Design review of the part built by this model. Coordinates are the model's own, in mm. Round coordinates to 2 decimals unless told otherwise and drop trailing zeros. Order: outer loops, then holes, each group sorted by start corner. A loop starts at its lowest first (then second) coordinate and runs counter-clockwise, first axis right, second up. Notation, with made-up numbers: M 32,-5.5 L 38,-5.5 A31 cw 38,25.5 Z; hole C -9,-34.5 d6. An arc over 180 degrees is marked long. Write each question's results on one line, items separated by ' | '. Start each with the question number.
Item 1: Wall thickness on line 1 (Z direction, x = -36, y = 0.55); line 2 (X direction, y = 0.5, z = -32); line 3 (Z direction, x = 43.5, y = 0.9): over which ranges is each line inside the solid? List them lowest first. Write a range as [from, to].
Item 2: Take a section at C-C, the plane y = 1.15. Count the separate pieces of the cut face and the enclosed holes in it, plus the area to 3 significant figures.
Item 3: Take a section at B-B, the plane z = 11.5. Write out the cut boundary in (x, y), plus the area to 3 significant figures.
Item 4: Take a section at A-A, the plane x = 43.5. Write out the cut boundary in (y, z), plus the area to 3 significant figures.
```python
from build123d import *

# Parameters (mm, degrees)
BOSS_EXTRUDE1_DEPTH = 2.3
SKETCH2_R           = 1
CUT_EXTRUDE1_DEPTH  = 2.3
SKETCH3_W           = 10
SKETCH3_H           = 2.3
CUT_EXTRUDE2_DEPTH  = 2.3
SKETCH4_W           = 15
SKETCH4_H           = 4
CUT_EXTRUDE3_DEPTH  = 10
SKETCH5_W           = 2.3
SKETCH5_H           = 10
CUT_EXTRUDE4_DEPTH  = 2.3
FILLET1_R           = 1
SKETCH6_W           = 4
SKETCH6_H           = 15
SKETCH6_W_2         = 10
SKETCH6_H_2         = 4
CUT_EXTRUDE5_DEPTH  = 10
FILLET3_R           = 1
SKETCH7_R           = 3
CUT_EXTRUDE6_DEPTH  = 10


with BuildPart() as part:
    # Sketch1 → Boss-Extrude1 (new body)
    with BuildSketch(Plane(origin=(0, 0, 0), x_dir=(1, 0, 0), z_dir=(0, 1, 0))):
        Polygon((0, -50), (-49.5, -50), (-49.5, 0), (-49.5, 35), (0, 35), (49.5, 35), (49.5, 0), (49.5, -50), align=None)
    extrude(amount=BOSS_EXTRUDE1_DEPTH)

    # Sketch2 → Cut-Extrude1 (cut)
    with BuildSketch(Plane(origin=(0, 2.3, 0), x_dir=(1, 0, 0), z_dir=(0, 1, 0))):
        with Locations((-20, 32)):
            Circle(SKETCH2_R)
        with Locations((20, 32)):
            Circle(SKETCH2_R)
    extrude(amount=-CUT_EXTRUDE1_DEPTH, mode=Mode.SUBTRACT)

    # Sketch3 → Cut-Extrude2 (cut)
    with BuildSketch(Plane(origin=(0, 2.3, 0), x_dir=(1, 0, 0), z_dir=(0, 1, 0))):
        with Locations((-15, -43.85)):
            Rectangle(SKETCH3_W, SKETCH3_H)
        with Locations((15, -43.85)):
            Rectangle(SKETCH3_W, SKETCH3_H)
    extrude(amount=-CUT_EXTRUDE2_DEPTH, mode=Mode.SUBTRACT)

    # Sketch4 → Cut-Extrude3 (cut)
    with BuildSketch(Plane(origin=(0, 2.3, 0), x_dir=(1, 0, 0), z_dir=(0, 1, 0))):
        with Locations((-17.5, 25)):
            Rectangle(SKETCH4_W, SKETCH4_H)
        with Locations((17.5, 25)):
            Rectangle(SKETCH4_W, SKETCH4_H)
    extrude(amount=-CUT_EXTRUDE3_DEPTH, mode=Mode.SUBTRACT)

    # Sketch5 → Cut-Extrude4 (cut)
    with BuildSketch(Plane(origin=(0, 2.3, 0), x_dir=(1, 0, 0), z_dir=(0, 1, 0))):
        with Locations((-36.15, 7.5)):
            Rectangle(SKETCH5_W, SKETCH5_H)
        with Locations((-36.15, -22.5)):
            Rectangle(SKETCH5_W, SKETCH5_H)
        with Locations((36.15, -22.5)):
            Rectangle(SKETCH5_W, SKETCH5_H)
        with Locations((36.15, 7.5)):
            Rectangle(SKETCH5_W, SKETCH5_H)
    extrude(amount=-CUT_EXTRUDE4_DEPTH, mode=Mode.SUBTRACT)

    # Fillet1
    fillet1_edges = [part.edges().sort_by_distance(p)[0] for p in [
        (-25, 1.15, -23),
        (-25, 1.15, -27),
        (-10, 1.15, -27),
        (-10, 1.15, -23),
        (10, 1.15, -23),
        (10, 1.15, -27),
        (25, 1.15, -27),
        (25, 1.15, -23),
    ]]
    fillet(fillet1_edges, radius=FILLET1_R)

    # Sketch6 → Cut-Extrude5 (cut)
    with BuildSketch(Plane(origin=(0, 2.3, 0), x_dir=(1, 0, 0), z_dir=(0, 1, 0))):
        with Locations((32.5, -7.5)):
            Rectangle(SKETCH6_W, SKETCH6_H)
        with Locations((-32.5, -7.5)):
            Rectangle(SKETCH6_W, SKETCH6_H)
        with Locations((-13, -38)):
            Rectangle(SKETCH6_W_2, SKETCH6_H_2)
        with Locations((13, -38)):
            Rectangle(SKETCH6_W_2, SKETCH6_H_2)
    extrude(amount=-CUT_EXTRUDE5_DEPTH, mode=Mode.SUBTRACT)

    # Fillet3
    fillet3_edges = [part.edges().sort_by_distance(p)[0] for p in [
        (-34.5, 1.15, 15),
        (-34.5, 1.15, 0),
        (-30.5, 1.15, 0),
        (-30.5, 1.15, 15),
        (34.5, 1.15, 15),
        (30.5, 1.15, 15),
        (30.5, 1.15, 0),
        (34.5, 1.15, 0),
        (-8, 1.15, 36),
        (-8, 1.15, 40),
        (-18, 1.15, 40),
        (-18, 1.15, 36),
        (8, 1.15, 40),
        (8, 1.15, 36),
        (18, 1.15, 36),
        (18, 1.15, 40),
    ]]
    fillet(fillet3_edges, radius=FILLET3_R)

    # Sketch7 → Cut-Extrude6 (cut)
    with BuildSketch(Plane(origin=(0, 2.3, 0), x_dir=(1, 0, 0), z_dir=(0, 1, 0))):
        with Locations((43.5, -42)):
            Circle(SKETCH7_R)
    extrude(amount=-CUT_EXTRUDE6_DEPTH, mode=Mode.SUBTRACT)


solid = part.part
```
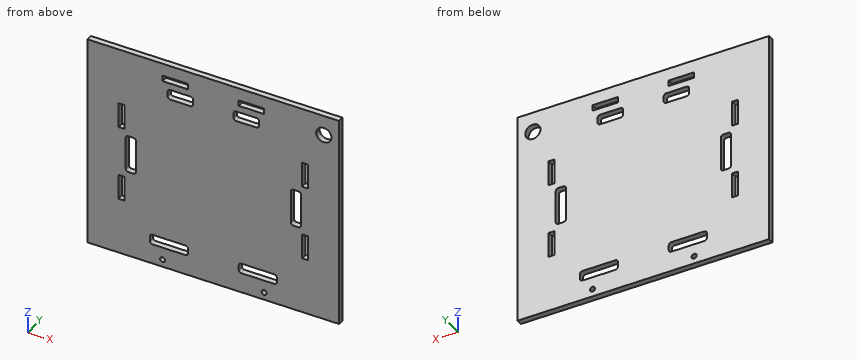
Results list:
1) line 1: [-35, -12.5], [-2.5, 17.5], [27.5, 50] | line 2: [-49.5, -21], [-19, 19], [21, 49.5] | line 3: [-35, 39], [45, 50]
2) separate pieces: 1 | enclosed holes: 15 | area: 7,930 mm²
3) outline: M -49.5,0 L -34.5,0 L -34.5,2.3 L -49.5,2.3 Z; M -30.5,0 L 30.5,0 L 30.5,2.3 L -30.5,2.3 Z; M 34.5,0 L 49.5,0 L 49.5,2.3 L 34.5,2.3 Z | area: 209 mm²
4) outline: M 0,-35 L 2.3,-35 L 2.3,39 L 0,39 Z; M 0,45 L 2.3,45 L 2.3,50 L 0,50 Z | area: 182 mm²
